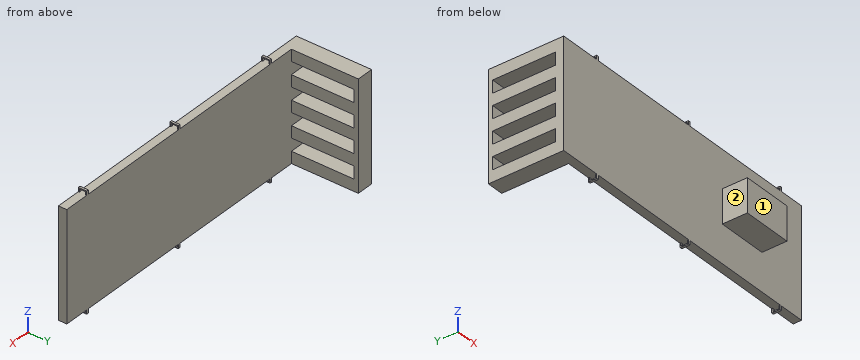
```python
from build123d import *

# Parameters (mm, degrees)
SKETCH1_W           = 914.4
SKETCH1_H           = 330.2
BOSS_EXTRUDE1_DEPTH = 25.4
SKETCH2_W           = 50.8
SKETCH2_H           = 330.2
BOSS_EXTRUDE2_DEPTH = 203.2
SKETCH5_W           = 6.35
SKETCH5_H           = 25.4
BOSS_EXTRUDE3_DEPTH = 12.7
SKETCH6_W           = 9.525
SKETCH6_H           = 19.05
CUT_EXTRUDE1_DEPTH  = 6.35
SKETCH7_W           = 9.525
SKETCH7_H           = 19.05
CUT_EXTRUDE2_DEPTH  = 6.35
SKETCH8_W           = 9.51738
SKETCH8_H           = 19.05
CUT_EXTRUDE3_DEPTH  = 6.35
SKETCH9_W           = 6.35
SKETCH9_H           = 25.4
BOSS_EXTRUDE4_DEPTH = 12.7
SKETCH10_W          = 9.525
SKETCH10_H          = 19.05
CUT_EXTRUDE4_DEPTH  = 6.35
SKETCH11_W          = 9.525
SKETCH11_H          = 19.05
CUT_EXTRUDE5_DEPTH  = 6.35
SKETCH12_W          = 9.525
SKETCH12_H          = 19.05
CUT_EXTRUDE6_DEPTH  = 6.35
SKETCH15_W          = 38.1
SKETCH15_H          = 190.5
CUT_EXTRUDE7_DEPTH  = 51.8
SKETCH16_W          = 152.4
SKETCH16_H          = 101.6
BOSS_EXTRUDE5_DEPTH = 76.2


with BuildPart() as part:
    # Sketch1 → Boss-Extrude1 (new body)
    with BuildSketch(Plane(origin=(0, 0, 0), x_dir=(1, 0, 0), z_dir=(0, 1, 0))):
        with Locations((457.2, -165.1)):
            Rectangle(SKETCH1_W, SKETCH1_H)
    extrude(amount=BOSS_EXTRUDE1_DEPTH)

    # Sketch2 → Boss-Extrude2 (add)
    with BuildSketch(Plane(origin=(0, 25.4, 0), x_dir=(1, 0, 0), z_dir=(0, 1, 0))):
        with Locations((25.4, -165.1)):
            Rectangle(SKETCH2_W, SKETCH2_H)
    extrude(amount=BOSS_EXTRUDE2_DEPTH)

    # Sketch5 → Boss-Extrude3 (add)
    with BuildSketch(Plane.XY.offset(330.2)):
        with Locations((130.175, 12.7)):
            Rectangle(SKETCH5_W, SKETCH5_H)
        with Locations((482.6, 12.7)):
            Rectangle(SKETCH5_W, SKETCH5_H)
        with Locations((835.025, 12.7)):
            Rectangle(SKETCH5_W, SKETCH5_H)
    extrude(amount=BOSS_EXTRUDE3_DEPTH)

    # Sketch6 → Cut-Extrude1 (cut)
    with BuildSketch(Plane(origin=(133.35, 0, 0), x_dir=(0, 0, -1), z_dir=(1, 0, 0))):
        with Locations((-334.9625, 12.7)):
            Rectangle(SKETCH6_W, SKETCH6_H)
    extrude(amount=-CUT_EXTRUDE1_DEPTH, mode=Mode.SUBTRACT)

    # Sketch7 → Cut-Extrude2 (cut)
    with BuildSketch(Plane(origin=(485.775, 0, 0), x_dir=(0, 0, -1), z_dir=(1, 0, 0))):
        with Locations((-334.9625, 12.7)):
            Rectangle(SKETCH7_W, SKETCH7_H)
    extrude(amount=-CUT_EXTRUDE2_DEPTH, mode=Mode.SUBTRACT)

    # Sketch8 → Cut-Extrude3 (cut)
    with BuildSketch(Plane(origin=(838.2, 0, 0), x_dir=(0, 0, -1), z_dir=(1, 0, 0))):
        with Locations((-334.95869, 12.7)):
            Rectangle(SKETCH8_W, SKETCH8_H)
    extrude(amount=-CUT_EXTRUDE3_DEPTH, mode=Mode.SUBTRACT)

    # Sketch9 → Boss-Extrude4 (add)
    with BuildSketch(Plane(origin=(0, 0, 0), x_dir=(-1, 0, 0), z_dir=(0, 0, -1))):
        with Locations((-835.025, 12.7)):
            Rectangle(SKETCH9_W, SKETCH9_H)
        with Locations((-482.6, 12.7)):
            Rectangle(SKETCH9_W, SKETCH9_H)
        with Locations((-130.175, 12.7)):
            Rectangle(SKETCH9_W, SKETCH9_H)
    extrude(amount=BOSS_EXTRUDE4_DEPTH)

    # Sketch10 → Cut-Extrude4 (cut)
    with BuildSketch(Plane(origin=(133.35, 0, 0), x_dir=(0, 0, -1), z_dir=(1, 0, 0))):
        with Locations((4.7625, 12.7)):
            Rectangle(SKETCH10_W, SKETCH10_H)
    extrude(amount=-CUT_EXTRUDE4_DEPTH, mode=Mode.SUBTRACT)

    # Sketch11 → Cut-Extrude5 (cut)
    with BuildSketch(Plane(origin=(485.775, 0, 0), x_dir=(0, 0, -1), z_dir=(1, 0, 0))):
        with Locations((4.7625, 12.7)):
            Rectangle(SKETCH11_W, SKETCH11_H)
    extrude(amount=-CUT_EXTRUDE5_DEPTH, mode=Mode.SUBTRACT)

    # Sketch12 → Cut-Extrude6 (cut)
    with BuildSketch(Plane(origin=(838.2, 0, 0), x_dir=(0, 0, -1), z_dir=(1, 0, 0))):
        with Locations((4.7625, 12.7)):
            Rectangle(SKETCH12_W, SKETCH12_H)
    extrude(amount=-CUT_EXTRUDE6_DEPTH, mode=Mode.SUBTRACT)

    # Sketch15 → Cut-Extrude7 (cut, through all)
    with BuildSketch(Plane(origin=(50.8, 0, 0), x_dir=(0, 0, -1), z_dir=(1, 0, 0))):
        with Locations((-275.59, 120.65)):
            Rectangle(SKETCH15_W, SKETCH15_H)
        with Locations((-201.93, 120.65)):
            Rectangle(SKETCH15_W, SKETCH15_H)
        with Locations((-128.27, 120.65)):
            Rectangle(SKETCH15_W, SKETCH15_H)
        with Locations((-54.61, 120.65)):
            Rectangle(SKETCH15_W, SKETCH15_H)
    extrude(amount=-CUT_EXTRUDE7_DEPTH, mode=Mode.SUBTRACT)

    # Sketch16 → Boss-Extrude5 (add)
    with BuildSketch(Plane.XZ):
        with Locations((685.8, 165.1)):
            Rectangle(SKETCH16_W, SKETCH16_H)
    extrude(amount=BOSS_EXTRUDE5_DEPTH)


solid = part.part
```
The listing builds one solid part. Answer for the finished solid, in the listing's coordinates (mm). Face numbers are marked on the shaded views. Coordinates: 2 decimals unless noted, no trailing zeros. Write each loop counter-clockwise with the first axis right and the second up, starting at its lowest first coordinate (ties: lowest second). Pieces come first, ordered by that corner, then holes. Notation, with made-up numbers: (-21.5, 26) - (19.5, 26) arc R20 ccw to (19.5, 53) - close; hole circle Ø9 at (-9, -27.5). An arc over 180 degrees is marked (long way). Return JSON: item names as keys, results as strings. Group by question number.
Q1. The part is cut by section A-A on z = 50. Write down the section's boundary in (x, y).
Q2. The part is cut by section C-C on z = 159. Write down the section's boundary in (x, y), and give its area (3 significant figures).
Q3. The part is cut by section D-D on x = 680. Write down the section's boundary in (y, z), and give its area (3 significant figures).
Q4. For a pull along Y with two mould halves and no side action, classify the marked faces 1 and 2 as +Y half, -Y half, draft (parallel to the pull), parting line (faces both ways), or undercut.
Q5. The part is cut by section B-B on y = 135. Write down the section's boundary in (x, z).
Q6. Find the intervals of material crossed by line 1 along Y through (x, z) = (827, 226.5); line 2 along Y through (x, z) = (673, 166.5); line 3 along Z through (x, y) = (687, -37.5), in increasing order. Write a range as [from, to].
Q7. Flat-ended cylindrical pins translate along their axes: pin 1 Ø19 at (x, z) = (25.5, 266.5) entering from -Y; pin 2 Ø6 at (y, z) = (117, 242.5) entering from -X; pin 3 Ø6.5 at (y, z) = (12, -6.5) entering from +X; pin 4 Ø10 at (x, y) = (476.5, 31) entering from -Z (1 decimal). Find the tip coordinate at first contact, or state that the pin passes through.
Evaluation:
{
 "1": {"outline": "(0, 0) - (914.4, 0) - (914.4, 25.4) - (0, 25.4) - close; (0, 215.9) - (50.8, 215.9) - (50.8, 228.6) - (0, 228.6) - close"},
 "2": {"outline": "(0, 0) - (609.6, 0) - (609.6, -76.2) - (762, -76.2) - (762, 0) - (914.4, 0) - (914.4, 25.4) - (50.8, 25.4) - (50.8, 228.6) - (0, 228.6) - close", "area": "45,200 mm2"},
 "3": {"outline": "(-76.2, 114.3) - (0, 114.3) - (0, 0) - (25.4, 0) - (25.4, 330.2) - (0, 330.2) - (0, 215.9) - (-76.2, 215.9) - close", "area": "16,100 mm2"},
 "4": {"face 1": "-Y half", "face 2": "draft"},
 "5": {"outline": "(0, 0) - (50.8, 0) - (50.8, 35.56) - (0, 35.56) - close; (0, 73.66) - (50.8, 73.66) - (50.8, 109.22) - (0, 109.22) - close; (0, 147.32) - (50.8, 147.32) - (50.8, 182.88) - (0, 182.88) - close; (0, 220.98) - (50.8, 220.98) - (50.8, 256.54) - (0, 256.54) - close; (0, 294.64) - (50.8, 294.64) - (50.8, 330.2) - (0, 330.2) - close"},
 "6": {"line 1": "y = [0, 25.4]", "line 2": "y = [-76.2, 25.4]", "line 3": "z = [114.3, 215.9]"},
 "7": {"pin 1": "stops at y = 0", "pin 2": "stops at x = 0", "pin 3": "stops at x = 838.2", "pin 4": "passes through"}
}
